Check sheet for the modelled part. Datum: model origin and axes. Units: mm. Give positions to 0.01 mm unless a question says otherwise; leave off trailing zeros. Write each loop counter-clockwise with the first axis right and the second up, starting at its lowest first coordinate (ties: lowest second). Pieces come first, ordered by that corner, then holes. Notation, with made-up numbers: M 36,12 L 61,12 A19 ccw 61,29 Z; hole C 79,-32.75 d7. An arc over 180 degrees is marked long. Use CSV: the item, a comma, the result in double quotes. Start each with the question number.
1. Cross-section at A-A, the plane x = -4. Enter the section's corners in (y, z) (3 decimals).
2. Depth check by flat-ended pin: P1, Ø1.5, axis at x = -0.5, y = 8.5, coming from the -Z side (3 decimals). Enter the tip coordinate at first touch or a pass-through.
3. Cross-section at C-C, the plane z = 667. Enter the section's corners in (x, y) (3 decimals), and give its area (3 significant figures).
4. Scan line: line 1 (Y direction, x = -5, z = 465) (3 decimals). Record every from-to range of solid material in increasing order.
Autodesk Inventor part; units mm, degrees
ref_plane "Start Plane" through (0, 0, -19.05) normal (0, 0, 1) x (1, 0, 0)
ref_plane "End Plane" through (0, 0, 781.05) normal (0, 0, 1) x (1, 0, 0)
ref_plane "Work Plane5" through (-50.8, 0, 781.05) normal (0, 0, 1) x (1, 0, 0)
ref_plane "Start Plane" through (0, 0, -19.05) normal (0, 0, 1) x (1, 0, 0)
ref_plane "End Plane" through (0, 0, 781.05) normal (0, 0, 1) x (1, 0, 0)
sketch "Sketch" plane through (0, 0, 0) normal (0, 0, 1) x (1, 0, 0)
  line L0 (-12.7, 12.7) -> (12.7, 12.7)
  line L1 (12.7, 12.7) -> (12.7, -12.7)
  line L2 (12.7, -12.7) -> (-12.7, -12.7)
  line L3 (-12.7, -12.7) -> (-12.7, 12.7)
  line L4 (9.525, 9.525) -> (-9.525, 9.525)
  line L5 (-9.525, 9.525) -> (-9.525, -9.525)
  line L6 (-9.525, -9.525) -> (9.525, -9.525)
  line L7 (9.525, -9.525) -> (9.525, 9.525)
  point P0 (0, 0)
  point P1 (0, 12.7)
  point P2 (-12.7, 0)
  dimension "width" = 25.4
  dimension "d1" = 3.175
extrude "Body" add sketch "Sketch" along normal up to surface (800.1 mm away) from surface at -19.05
sketch "Sketch4" plane through (0, 0, 0) normal (0, 0, 1) x (1, 0, 0)
  line L0 (0, 0) -> (10, 0)
ref_plane "Work Plane4" through (0, 0, 0) normal (0, -1, 0) x (1, 0, 0)
sketch "Sketch5" plane through (0, 0, 0) normal (0, -1, 0) x (1, 0, 0)
  line L0 (-2, -19.05) -> (12, -19.05)
  line L1 (-2, 781.05) -> (12, 781.05)
  dimension "d9" = 800.1
ref_plane "Work Plane5" through (-50.8, 0, 781.05) normal (0, 0, 1) x (1, 0, 0)
split "Split1" plane through (-50.8, 0, 781.05) removes the side toward (0, 0, 1)
ref_plane "Work Plane6" through (-12.7, 0, -19.05) normal (0, 0, -1) x (-1, 0, 0)
split "Split2" plane through (-12.7, 0, -19.05) removes the side toward (0, 0, -1)
equation "\"G_OFFSET_START\" = 19.05"
equation "\"G_OFFSET_END\" = 19.05"
equation "\"d4\" = -G_OFFSET_START"
equation "\"d5\" = length + G_OFFSET_END"
equation "\"G_L\" = 762"
properties part number "Square Tube Profile" material "Aluminum-6061"
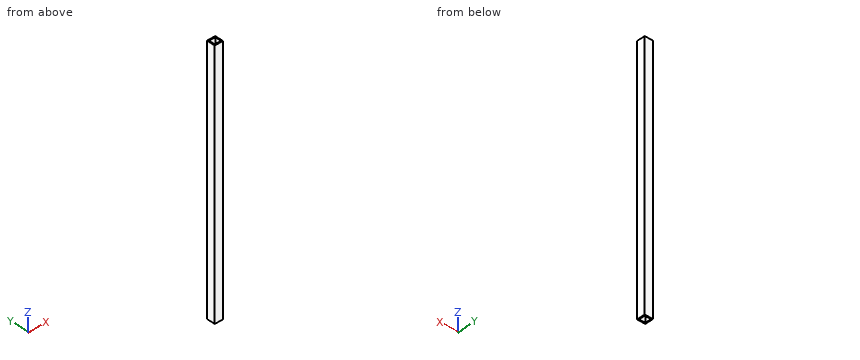
Worked answers:
1,outline,"M -12.7,-19.05 L -9.525,-19.05 L -9.525,781.05 L -12.7,781.05 Z; M 9.525,-19.05 L 12.7,-19.05 L 12.7,781.05 L 9.525,781.05 Z"
2,P1,"passes through"
3,outline,"M -12.7,-12.7 L 12.7,-12.7 L 12.7,12.7 L -12.7,12.7 Z; hole M -9.525,-9.525 L 9.525,-9.525 L 9.525,9.525 L -9.525,9.525 Z"
3,area,"282 mm^2"
4,line 1,"y = -12.7 to -9.525, 9.525 to 12.7"
